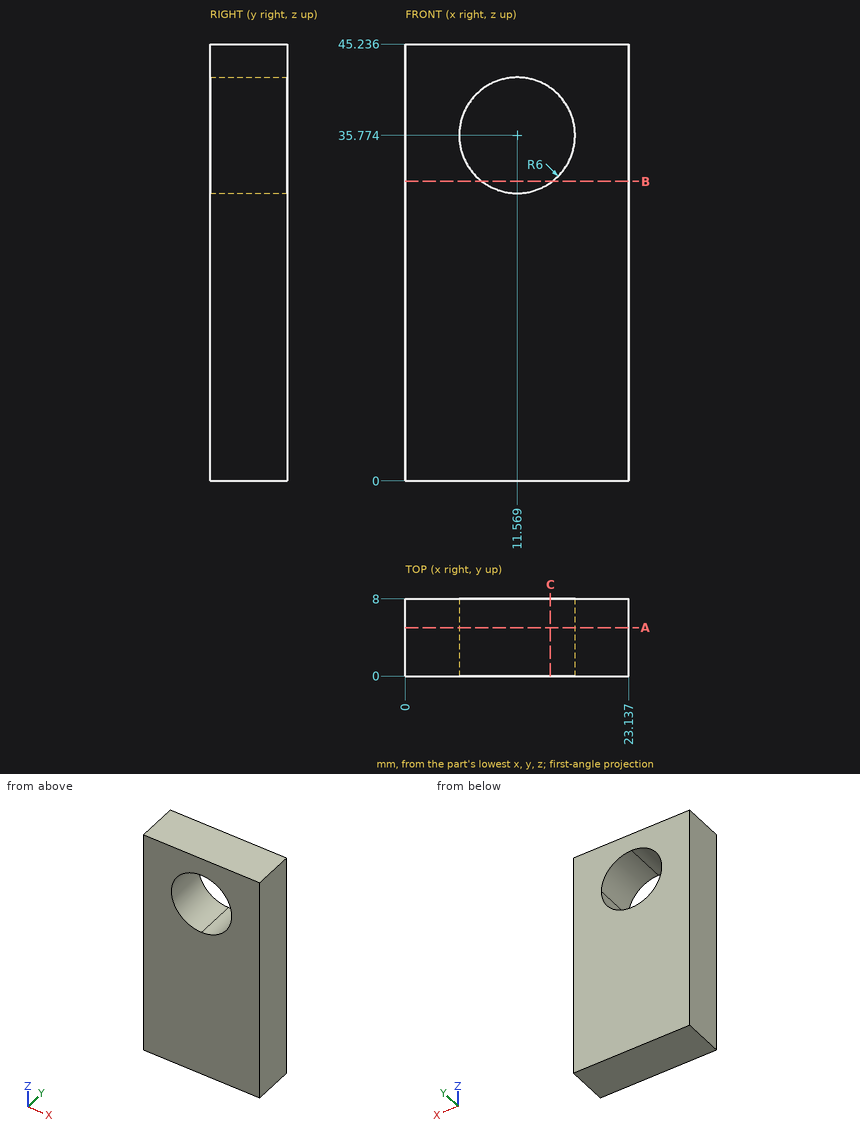
Input: dimensioned drawing with shaded views. Units: mm. Origin: part minimum x, y, z. Round coordinates to 2 decimals unless told otherwise and drop trailing zeros. Order: outer loops, then holes, each group sorted by start corner. A loop starts at its lowest first (then second) coordinate and runs counter-clockwise, first axis right, second up.
Q1. Section A-A, the plane y = 5. Output: boundary loops of the cut face in (x, z).
Result sheet:
outline: (0, 0) - (23.14, 0) - (23.14, 45.24) - (0, 45.24) - close; hole circle Ø12 at (11.57, 35.77)
Q2. Section B-B, the plane z = 31. Output: boundary loops of the cut face in (x, y).
Result sheet:
outline: (0, 0) - (7.93, 0) - (7.93, 8) - (0, 8) - close; (15.2, 0) - (23.14, 0) - (23.14, 8) - (15.2, 8) - close
Q3. Material intervals for probe 1 along X at (y, z) = (4.75, 36) (1 decimal); probe 2 along Z at (x, y) = (11.5, 1.25) (1 decimal); probe 3 along X at (y, z) = (5, 41) (1 decimal), sorted ascending.
Result sheet:
probe 1: x = 0 to 5.6, 17.6 to 23.1
probe 2: z = 0 to 29.8, 41.8 to 45.2
probe 3: x = 0 to 8.6, 14.5 to 23.1
Q4. Section C-C, the plane x = 15. Output: boundary loops of the cut face in (y, z) (1 decimal), and give its area (3 significant figures).
Result sheet:
outline: (0, 0) - (8, 0) - (8, 30.9) - (0, 30.9) - close; (0, 40.7) - (8, 40.7) - (8, 45.2) - (0, 45.2) - close
area: 283 mm2
